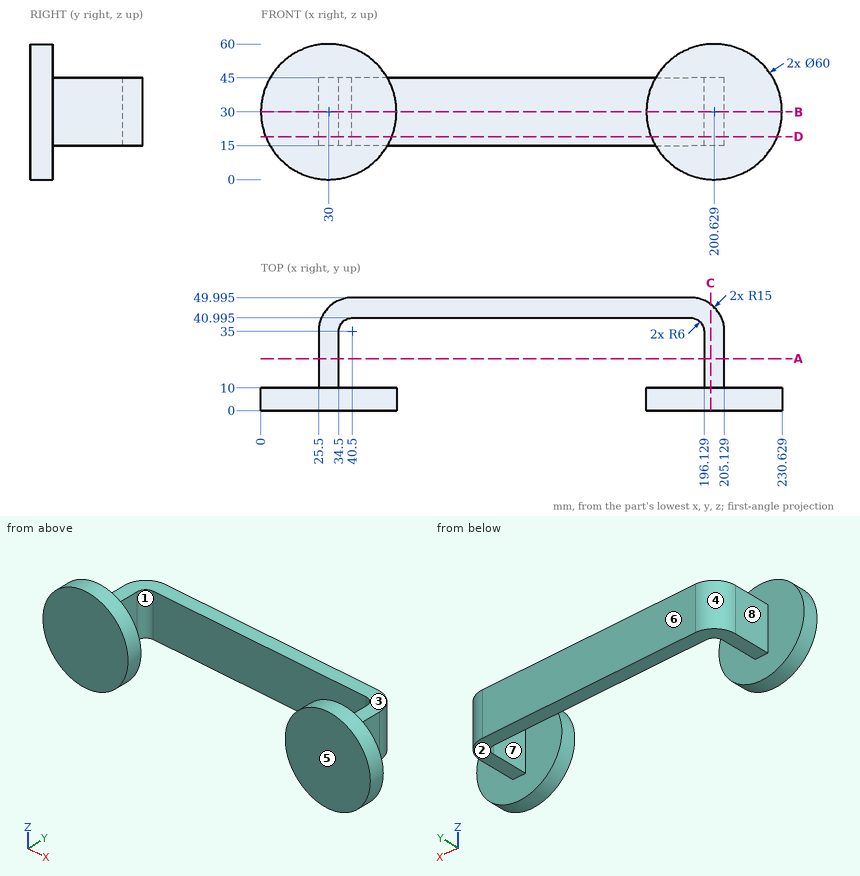
Job drawing, mm, ordinate dimensions from the low corner. One solid piece. A direction names the side the tool comes from. Round coordinates to 2 decimals unless told otherwise and drop trailing zeros. Write each loop counter-clockwise with the first axis right and the second up, starting at its lowest first coordinate (ties: lowest second). Pieces come first, ordered by that corner, then holes. Notation, with made-up numbers: (68, 14.25) -> (127, 14.25) arc R10 cw to (127, 22.25) -> close; hole circle Ø3 at (22, -19). An arc over 180 degrees is marked (long way). Answer as a JSON object with one key per item and string values.
(1) Probe probe 1 along Y at (x, z) = (184, 33) (1 decimal); probe 2 along X at (y, z) = (25.5, 36); probe 3 along Y at (x, z) = (116, 34) (1 decimal). List the from-to ranges inside material, lowest first. Write a range as [from, to].
Reported:
{"probe 1": "y = [0, 10], [41, 50]", "probe 2": "x = [25.5, 34.5], [196.13, 205.13]", "probe 3": "y = [41, 50]"}
(2) Pin check, flat tips, straight feed: P1, Ø12.5, axis at y = 19.5, z = 26, coming from the -X side; P2, Ø5, axis at y = 26, z = 32.5, coming from the +X side; P3, Ø20, axis at y = 18.5, z = 25.5, coming from the -X side; P4, Ø20, axis at x = 98, y = 38.5, coming from the -Z side. Stop position of each tip, or through.
Reported:
{"P1": "stops at x = 25.5", "P2": "stops at x = 205.13", "P3": "stops at x = 0", "P4": "stops at z = 15"}
(3) Band-saw the part on A-A, the plane y = 23. List the corners of the cut face in (x, z), then the cut area to 3 significant figures.
Reported:
{"outline": "(25.5, 15) -> (34.5, 15) -> (34.5, 45) -> (25.5, 45) -> close; (196.13, 15) -> (205.13, 15) -> (205.13, 45) -> (196.13, 45) -> close", "area": "540 mm^2"}
(4) Band-saw the part on D-D, the plane z = 19. List the corners of the cut face in (x, y) (1 decimal), then the cut area to 3 significant figures.
Reported:
{"outline": "(2.1, 0) -> (57.9, 0) -> (57.9, 10) -> (34.5, 10) -> (34.5, 35) arc R6 cw to (40.3, 41) -> (190.1, 41) arc R6 cw to (196.1, 35) -> (196.1, 10) -> (172.7, 10) -> (172.7, 0) -> (228.5, 0) -> (228.5, 10) -> (205.1, 10) -> (205.1, 35) arc R15 ccw to (190.1, 50) -> (40.1, 50) arc R15 ccw to (25.5, 35) -> (25.5, 10) -> (2.1, 10) -> close", "area": "3,210 mm^2"}
(5) Which spindle directions (+Z, -Z, +X, -X, +Y, -Y) get a long thin tool onto all of the face, cutting with end or side? Do the marked faces 1, 2, 3, 4 and 5. Say none if no direction does.
Reported:
{"face 1": "+Z, -Z", "face 2": "-Z, +X, -X, +Y", "face 3": "+Z, +X, -X, +Y", "face 4": "+Z, -Z, -X, +Y", "face 5": "+Z, -Z, +X, -X, -Y"}
(6) Band-saw the part on C-C, the plane x = 199. List the corners of the cut face in (y, z) (1 decimal).
Reported:
{"outline": "(0, 0) -> (10, 0) -> (10, 15) -> (47.1, 15) -> (47.1, 45) -> (10, 45) -> (10, 60) -> (0, 60) -> close"}
(7) Band-saw the part on B-B, the plane z = 30. List the corners of the cut face in (x, y) (1 decimal), then the cut area to 3 significant figures.
Reported:
{"outline": "(0, 0) -> (60, 0) -> (60, 10) -> (34.5, 10) -> (34.5, 35) arc R6 cw to (40.3, 41) -> (190.1, 41) arc R6 cw to (196.1, 35) -> (196.1, 10) -> (170.6, 10) -> (170.6, 0) -> (230.6, 0) -> (230.6, 10) -> (205.1, 10) -> (205.1, 35) arc R15 ccw to (190.1, 50) -> (40.1, 50) arc R15 ccw to (25.5, 35) -> (25.5, 10) -> (0, 10) -> close", "area": "3,290 mm^2"}
(8) Two-plate mould, pull along X, no slides. Class the marked faces 6, 7 and 8: +X half, -X half, draft (parallel to the pull), parting line (faces both ways), or undercut.
Reported:
{"face 6": "draft", "face 7": "undercut", "face 8": "-X half"}
